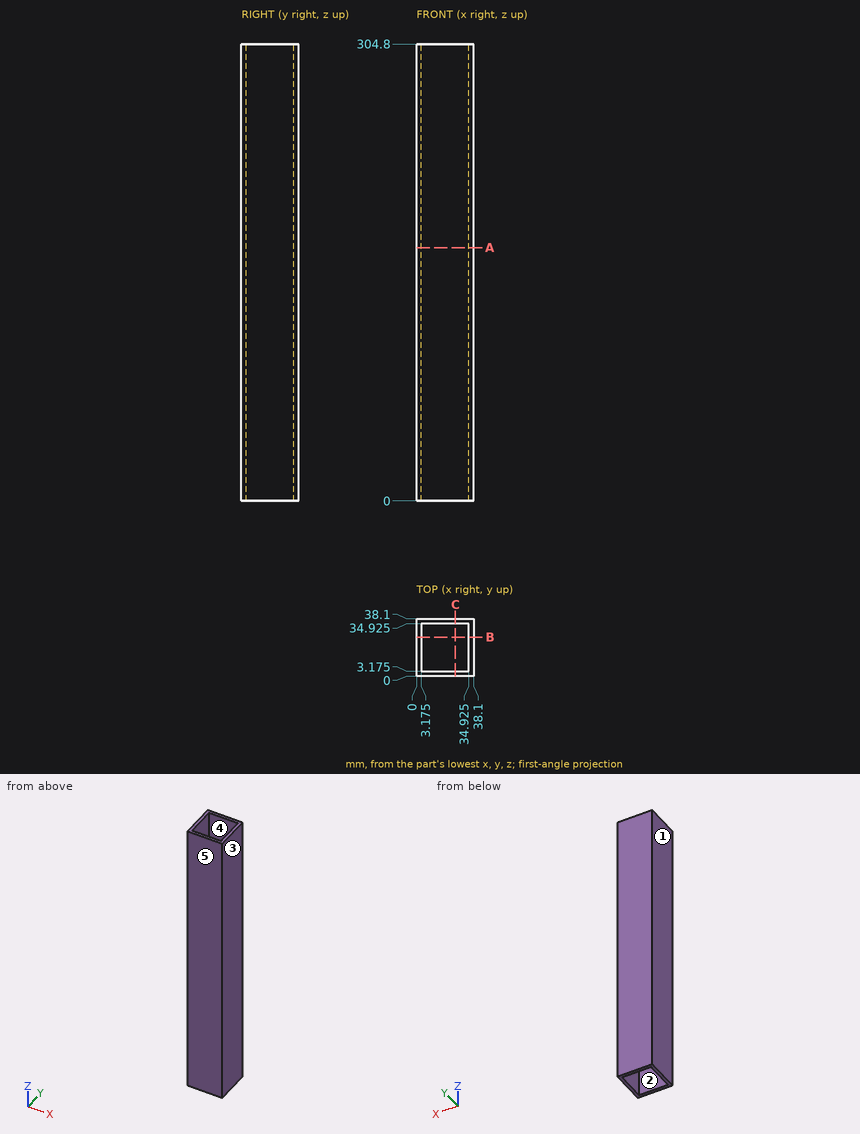
For this review, use the dimensioned drawing (mm, ordinates from the lowest corner) and the shaded views. A direction names the side the tool comes from. Give positions to 0.01 mm unless a question says otherwise; leave off trailing zeros. Order: outer loops, then holes, each group sorted by start corner. A loop starts at its lowest first (then second) coordinate and runs counter-clockwise, first axis right, second up. Notation, with made-up numbers: M 1,10.25 L 31,10.25 A21 ccw 31,27.25 Z; hole C -1.5,42 d2. An arc over 180 degrees is marked long. Use one line per item in the form item = value. Start each with the question number.
Item 1: Insertion check: pin 1 Ø8 at (x, y) = (7.5, 11) entering from -Z. The pin has a flat end and moves straight along its axis. Give the tip position at first contact, or say it passes through.
Item 2: For the marked faces 4 and 5, list the 3-axis set-ups (+Z, -Z, +X, -X, +Y, -Y) from which the entire face can be reached by the end or side of a thin tool; tool diameter is ignored.
Item 3: To check wall thickness, follow line 1 along X through (y, z) = (27.5, 221) (3 decimals). State the ranges of the line that lie inside material, in increasing order. Write a range as from..to.
Item 4: We need section A-A on z = 169. Give the boundary of the cut face in (x, y) (3 decimals), plus the area to 3 significant figures.
Item 5: We need section B-B on y = 26. Give the boundary of the cut face in (x, z) (3 decimals).
Item 6: The part is to be moulded in two halves that separate along X. For the marked faces 1, 2 and 3, say which applies: pulls with the +X half, pulls with the -X half, needs draft (parallel to the pull), parting line crosses it, or undercut.
Completed:
q1.pin_1 = through
q2.face_4 = +Z, -Z
q2.face_5 = +Z, -Z, +X, -X, -Y
q3.line_1 = 0..3.175, 34.925..38.1
q4.outline = M 0,0 L 38.1,0 L 38.1,38.1 L 0,38.1 Z; hole M 3.175,3.175 L 34.925,3.175 L 34.925,34.925 L 3.175,34.925 Z
q4.area = 444 mm²
q5.outline = M 0,0 L 3.175,0 L 3.175,304.8 L 0,304.8 Z; M 34.925,0 L 38.1,0 L 38.1,304.8 L 34.925,304.8 Z
q6.face_1 = pulls with the -X half
q6.face_2 = undercut
q6.face_3 = pulls with the +X half
